Model file for the job. Use its own axes, mm. Face numbers are marked on the shaded views. A direction names the side the tool comes from. Round coordinates to 2 decimals unless told otherwise and drop trailing zeros. Order: outer loops, then holes, each group sorted by start corner. A loop starts at its lowest first (then second) coordinate and runs counter-clockwise, first axis right, second up. Notation, with made-up numbers: (-21, -26.75) -> (21, -26.75) arc R30 cw to (21, -0.75) -> close; hole circle Ø5 at (-9, 24.5). An arc over 180 degrees is marked (long way). Answer as CSV lines item,"result".
```python
from build123d import *

# Parameters (mm, degrees)
SKETCH1_W           = 108.64
SKETCH1_H           = 26
SKETCH1_R           = 1
SKETCH1_R_2         = 2.75
BOSS_EXTRUDE1_DEPTH = 2
CUT_EXTRUDE2_REACH  = 4
SKETCH5_R           = 2
SKETCH3_W           = 15
SKETCH3_H           = 3
BOSS_EXTRUDE2_DEPTH = 20
SKETCH4_R           = 2.1
CUT_EXTRUDE1_DEPTH  = 15


with BuildPart() as part:
    # Sketch1 → Boss-Extrude1 (new body)
    with BuildSketch(Plane.XY):
        with Locations((54.32, 13)):
            Rectangle(SKETCH1_W, SKETCH1_H)
        with Locations((30.82, 21)):
            Circle(SKETCH1_R, mode=Mode.SUBTRACT)
        with Locations((30.82, 5)):
            Circle(SKETCH1_R, mode=Mode.SUBTRACT)
        with Locations((77.82, 13)):
            Circle(SKETCH1_R, mode=Mode.SUBTRACT)
        with Locations((10, 13)):
            Circle(SKETCH1_R_2, mode=Mode.SUBTRACT)
        with Locations((98.64, 13)):
            Circle(SKETCH1_R_2, mode=Mode.SUBTRACT)
    extrude(amount=BOSS_EXTRUDE1_DEPTH)

    # Sketch5 → Cut-Extrude2 (cut, up to next)
    with BuildSketch(Plane.XY.offset(2), mode=Mode.PRIVATE) as cut_extrude2_sk1:
        with Locations((26, 1.043474904)):
            Circle(SKETCH5_R)
    cut_extrude2_tool1 = extrude(cut_extrude2_sk1.sketch, amount=-CUT_EXTRUDE2_REACH, mode=Mode.PRIVATE) & part.part
    add(cut_extrude2_tool1.solids().sort_by_distance((26, 1.043475, 2))[0], mode=Mode.SUBTRACT)
    # Sketch5 → Cut-Extrude2 (cut, up to next)
    with BuildSketch(Plane.XY.offset(2), mode=Mode.PRIVATE) as cut_extrude2_sk2:
        with Locations((82.64, 1.043474904)):
            Circle(SKETCH5_R)
    cut_extrude2_tool2 = extrude(cut_extrude2_sk2.sketch, amount=-CUT_EXTRUDE2_REACH, mode=Mode.PRIVATE) & part.part
    add(cut_extrude2_tool2.solids().sort_by_distance((82.64, 1.043475, 2))[0], mode=Mode.SUBTRACT)

    # Sketch3 → Boss-Extrude2 (add)
    with BuildSketch(Plane.XY.offset(2)):
        with Locations((74.14, 24.5)):
            Rectangle(SKETCH3_W, SKETCH3_H)
    extrude(amount=BOSS_EXTRUDE2_DEPTH)

    # Sketch4 → Cut-Extrude1 (cut)
    with BuildSketch(Plane(origin=(0, 26, 0), x_dir=(1, 0, 0), z_dir=(0, 1, 0))):
        with Locations((74.32, -18)):
            Circle(SKETCH4_R)
    extrude(amount=-CUT_EXTRUDE1_DEPTH, mode=Mode.SUBTRACT)


solid = part.part
```
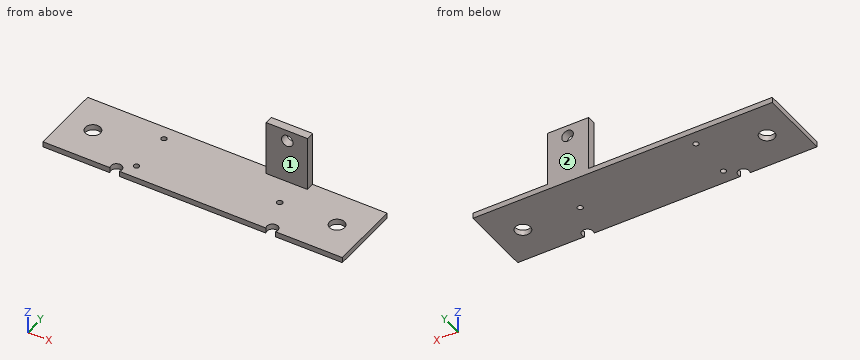
Q1. Tool access for the marked faces 1 and 2: list every direction of +Z, -Z, +X, -X, +Y, -Y with a clear straight run to the whole face (end or side of a thin tool).
Checks:
face 1,"+Z, +X, -X, -Y"
face 2,"+Z, -Z, +X, -X, +Y"
Q2. Saw through at A-A (y = 5). Write the cut outline in (x, z).
Checks:
outline,"(0, 0) -> (29.82, 0) -> (29.82, 2) -> (0, 2) -> close; (31.82, 0) -> (108.64, 0) -> (108.64, 2) -> (31.82, 2) -> close"
Q3. Flat gauge pins, fed straight in: pin 1 (2.5 mm diameter, centred on y = 24.5, z = 10, fed in from -X); pin 2 (12 mm diameter, centred on x = 71.5, z = 11, fed in from -Y); pin 3 (6.5 mm diameter, centred on x = 26, y = 1.04, fed in from +Z); pin 4 (1 mm diameter, centred on x = 41.5, y = 7, fed in from -Z). Where does each tip first touch, or does it go through?
Checks:
pin 1,"x = 66.64"
pin 2,"y = 23"
pin 3,"z = 2"
pin 4,"z = 0"
Q4. Wall check: L1, parallel to Y at x = 30.82, z = 0.7; L2, parallel to Y at x = 77.82, z = 1.1; L3, parallel to X at y = 24.5, z = 18. Give the ranges that are in metal, low to high. Write a range as [from, to].
Checks:
L1,"[0, 4], [6, 20], [22, 26]"
L2,"[0, 12], [14, 26]"
L3,"[66.64, 72.22], [76.42, 81.64]"
Q5. Saw through at D-D (x = 10). Write the cut outline in (y, z), plus the area to 3 significant figures.
Checks:
outline,"(0, 0) -> (10.25, 0) -> (10.25, 2) -> (0, 2) -> close; (15.75, 0) -> (26, 0) -> (26, 2) -> (15.75, 2) -> close"
area,"41.0 mm²"
Q6. Saw through at C-C (y = 13). Write the cut outline in (x, z).
Checks:
outline,"(0, 0) -> (7.25, 0) -> (7.25, 2) -> (0, 2) -> close; (12.75, 0) -> (76.82, 0) -> (76.82, 2) -> (12.75, 2) -> close; (78.82, 0) -> (95.89, 0) -> (95.89, 2) -> (78.82, 2) -> close; (101.39, 0) -> (108.64, 0) -> (108.64, 2) -> (101.39, 2) -> close"
Q7. Saw through at B-B (x = 74.32). Write the cut outline in (y, z).
Checks:
outline,"(0, 0) -> (26, 0) -> (26, 15.9) -> (23, 15.9) -> (23, 2) -> (0, 2) -> close; (23, 20.1) -> (26, 20.1) -> (26, 22) -> (23, 22) -> close"
